Source: CAD feature listing. Evaluate the final solid. Frame: model axes, mm. Face numbers are marked on the shaded views. A direction names the side the tool comes from. Give positions to 0.01 mm unless a question says otherwise; leave off trailing zeros. Loops run counter-clockwise (first coordinate to the right, second up) from the corner with the lowest first, then second, coordinate; pieces in that order, holes last. Notation, with made-up numbers: M -10,1 L 33,1 A29 ccw 33,25 Z; hole C -39.75,36 d2. An arc over 180 degrees is marked long. Answer in a Markdown table with one row per item.
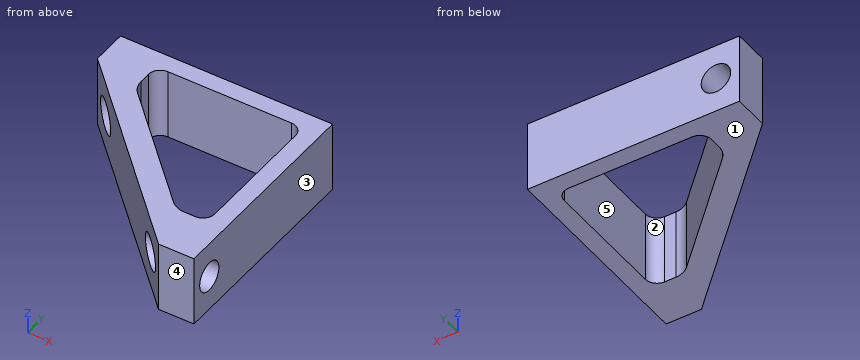
```python
from build123d import *

# Parameters (mm, degrees)
EXTRUDE_1_DEPTH     = 6
CUT_EXTRUDE_1_DEPTH = 27.153393661
SKETCH_3_R          = 1.25
CUT_EXTRUDE_2_DEPTH = 27.153393661
FILLET_1_R          = 1
FILLET_2_R          = 1.75


with BuildPart() as part:
    # 草图1 → 凸台-拉伸1 (new body)
    with BuildSketch(Plane.XY):
        Polygon((-18, 0), (0, 0), (0, -18), (-3, -18), (-18, -3), align=None)
    extrude(amount=EXTRUDE_1_DEPTH)

    # 草图2 → 切除-拉伸1 (cut, through all)
    with BuildSketch(Plane.XY.offset(6)):
        Polygon((-14, -1.5), (-14, -4.171572875), (-4.171572875, -14), (-1.5, -14), (-1.5, -1.5), align=None)
    extrude(amount=-CUT_EXTRUDE_1_DEPTH, mode=Mode.SUBTRACT)

    # 草图3 → 切除-拉伸2 (cut, through all)
    with BuildSketch(Plane(origin=(0, 0, 0), x_dir=(0, 0, -1), z_dir=(1, 0, 0))):
        with Locations(Location((-3, -16, 0), (0, 0, 90))):
            Circle(SKETCH_3_R)
    cut_extrude_2 = extrude(amount=-CUT_EXTRUDE_2_DEPTH, mode=Mode.SUBTRACT)

    # 镜向1: 切除-拉伸2 across plane
    add(cut_extrude_2.mirror(Plane(origin=(0, 0, 0), x_dir=(0, 0, 1), z_dir=(-0.7071067811865476, 0.7071067811865475, 0))), mode=Mode.SUBTRACT)

    # 圆角1
    fillet_1_edges = [part.edges().sort_by_distance(p)[0] for p in [
        (-1.5, -14, 3),
        (-14, -1.5, 3),
        (-1.5, -1.5, 3),
    ]]
    fillet(fillet_1_edges, radius=FILLET_1_R)

    # 圆角2
    fillet_2_edges = [part.edges().sort_by_distance(p)[0] for p in [
        (-4.171572875, -14, 3),
        (-14, -4.171572875, 3),
    ]]
    fillet(fillet_2_edges, radius=FILLET_2_R)


solid = part.part
```
Q1. Contact query for a flat-ended pin moving along its axis: pin 1 Ø3 at (y, z) = (-8.5, 2) entering from -X. Output: stop coordinate, or through.
Values follow:
| item | result |
|---|---|
| pin 1 | x = -14 |
Q2. Section query C-C (y = -2). Output: boundary loops of the cut face in (x, z), plus the area to 3 significant figures.
Values follow:
| item | result |
|---|---|
| outline | M -18,0 L -13.87,0 L -13.87,6 L -18,6 Z; M -1.63,0 L 0,0 L 0,6 L -1.63,6 Z; hole C -16,3 d2.5 |
| area | 29.7 mm^2 |
Q3. Section query A-A (x = -16.75). Output: boundary loops of the cut face in (y, z), plus the area to 3 significant figures.
Values follow:
| item | result |
|---|---|
| outline | M -4.25,0 L 0,0 L 0,2 L -4.25,2 Z; M -4.25,4 L 0,4 L 0,6 L -4.25,6 Z |
| area | 17.0 mm^2 |
Q4. Section query B-B (z = 3). Output: boundary loops of the cut face in (x, y), plus the area to 3 significant figures.
Values follow:
| item | result |
|---|---|
| outline | M -18,-3 L -17.25,-3.75 L -17.25,0 L -18,0 Z; M -14.75,-6.25 L -6.25,-14.75 L 0,-14.75 L 0,0 L -14.75,0 Z; M -3.75,-17.25 L -3,-18 L 0,-18 L 0,-17.25 Z; hole M -14,-3.45 A1.75 ccw -13.49,-4.68 L -4.68,-13.49 A1.75 ccw -3.45,-14 L -2.5,-14 A1 ccw -1.5,-13 L -1.5,-2.5 A1 ccw -2.5,-1.5 L -13,-1.5 A1 ccw -14,-2.5 Z |
| area | 79.3 mm^2 |
Q5. Section query D-D (y = -16). Output: boundary loops of the cut face in (x, z), plus the area to 3 significant figures.
Values follow:
| item | result |
|---|---|
| outline | M -5,0 L 0,0 L 0,1.75 L -5,1.75 Z; M -5,4.25 L 0,4.25 L 0,6 L -5,6 Z |
| area | 17.5 mm^2 |
Q6. Ray query, probe 1 along Z at (x, y) = (-16, -3); probe 2 along Y at (x, z) = (-2.5, 2.25); probe 3 along X at (y, z) = (-2.5, 3). Return the intervals inside material, ascending. Write a range as from..to.
Values follow:
| item | result |
|---|---|
| probe 1 | 0..1.75, 4.25..6 |
| probe 2 | -18..-17, -15..-14, -1.5..0 |
| probe 3 | -18..-17.25, -14.75..-14, -1.5..0 |
Q7. Reachability of the marked faces 1 and 2 from +Z, -Z, +X, -X, +Y, -Y: full face, straight path, thin tool, end or side. Return the list, or none.
Values follow:
| item | result |
|---|---|
| face 1 | -Z, +X, -X, +Y, -Y |
| face 2 | +Z, -Z |
Q8. Mould query, pull axis X, two halves, no side actions, for the marked faces 3, 4 and 5. Classes: +X half, -X half, draft (parallel to the pull), parting line (faces both ways), or undercut.
Values follow:
| item | result |
|---|---|
| face 3 | +X half |
| face 4 | draft |
| face 5 | undercut |
